Could you check a few things on this drawing? It's one solid part, dimensions in mm from its lowest x, y, z. Coordinates: 2 decimals unless noted, no trailing zeros. Write each loop counter-clockwise with the first axis right and the second up, starting at its lowest first coordinate (ties: lowest second). Pieces come first, ordered by that corner, then holes.
Item 1: I want a section at A-A (x = 402.5). Please give me the cut outline in (y, z), and give its area (3 significant figures).
Item 2: I'm going to push flat-ended pins straight in: P1, Ø2, axis at y = 2.5, z = 52, coming from the +X side (1 decimal); P2, Ø3, axis at y = 6.5, z = 243, coming from the -X side; P3, Ø1.5, axis at y = 2.5, z = 318.5, coming from the +X side. Where does each tip first touch, or does it pass through?
Item 3: I want a section at C-C (z = 204.5). Please give me the cut outline in (x, y), and give its area (3 significant figures).
Item 4: I want a section at B-B (y = 2.75). Please give me the cut outline in (x, z), and give its area (3 significant figures).
Item 5: Please list where these lines run through material, in increasing order: line 1 (X direction, y = 3.5, z = 249); line 2 (Z direction, x = 365, y = 0.5) (1 decimal); line 3 (X direction, y = 2.25, z = 382.5) (1 decimal).
Item 6: I want a section at D-D (x = 210). Please give me the cut outline in (y, z), and give its area (3 significant figures).
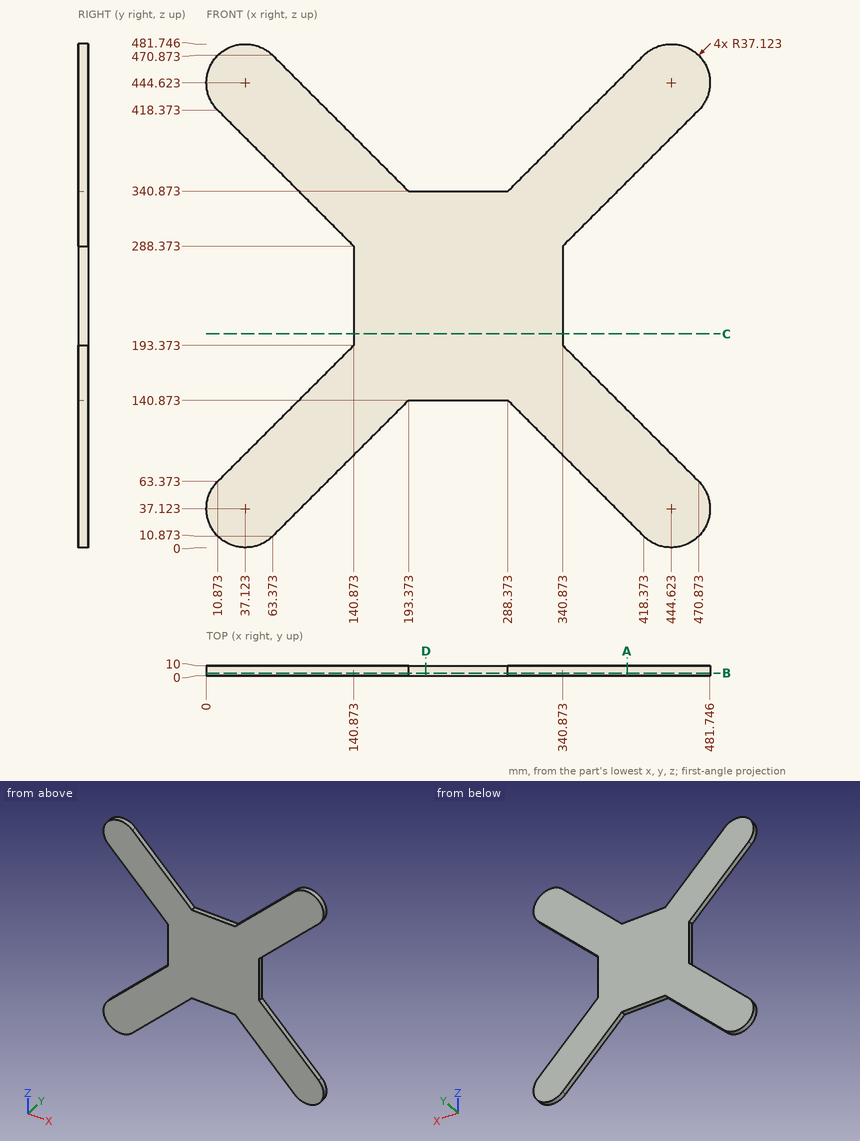
Answer:
1. outline: (0, 26.75) - (10, 26.75) - (10, 131.75) - (0, 131.75) - close; (0, 350) - (10, 350) - (10, 455) - (0, 455) - close
1. area: 2,100 mm2
2. P1: stops at x = 479.1
2. P2: stops at x = 140.87
2. P3: stops at x = 371.75
3. outline: (140.87, 0) - (340.87, 0) - (340.87, 10) - (140.87, 10) - close
3. area: 2,000 mm2
4. outline: (10.87, 63.37) arc R37.12 ccw to (63.37, 10.87) - (193.37, 140.87) - (288.37, 140.87) - (418.37, 10.87) arc R37.12 ccw to (470.87, 63.37) - (340.87, 193.37) - (340.87, 288.37) - (470.87, 418.37) arc R37.12 ccw to (418.37, 470.87) - (288.37, 340.87) - (193.37, 340.87) - (63.37, 470.87) arc R37.12 ccw to (10.87, 418.37) - (140.87, 288.37) - (140.87, 193.37) - close
4. area: 97,700 mm2
5. line 1: x = 140.87 to 340.87
5. line 2: z = 64.2 to 169.2, 312.5 to 417.5
5. line 3: x = 46.7 to 151.7, 330 to 435
6. outline: (0, 140.87) - (10, 140.87) - (10, 340.87) - (0, 340.87) - close
6. area: 2,000 mm2
